```python
from build123d import *

# Parameters (mm, degrees)
BOSS_EXTRU_1_DEPTH      = 50
ESQUISSE3_R             = 25
BOSS_EXTRU_2_DEPTH      = 10
ESQUISSE4_R             = 25
BOSS_EXTRU_3_DEPTH      = 15
COQUE2_START            = 3
COQUE2_DEPTH            = 44
ESQUISSE6_R             = 2.5
ENL_V_MAT_EXTRU_1_DEPTH = 109.272397717


with BuildPart() as part:
    # Esquisse1 → Boss.-Extru.1 (new body)
    with BuildSketch(Plane.XY):
        Polygon((-31.809910954, -22.428852102), (-16.234936413, -34.975571516), (33.765063587, -34.975571516), (62.690506023, -0.503571576), (54.008097139, 48.736816075), (33.432510355, 62.937000175), (-31.809910954, 37.571147898), align=None)
    extrude(amount=BOSS_EXTRU_1_DEPTH)

    # Esquisse3 → Boss.-Extru.2 (add)
    with BuildSketch(Plane(origin=(60.714040151, 10.705523386, 0), x_dir=(0, 0, -1), z_dir=(0.9848077530122085, 0.17364817766692822, 0))):
        with Locations(Location((-25, 13.61798668, 0), (0, 0, 90))):
            Circle(ESQUISSE3_R)
    extrude(amount=BOSS_EXTRU_2_DEPTH)

    # Esquisse4 → Boss.-Extru.3 (add, symmetric)
    with BuildSketch(Plane.ZY.offset(31.809910954)):
        with Locations((25, -3.702211809)):
            Circle(ESQUISSE4_R)
    extrude(amount=BOSS_EXTRU_3_DEPTH, both=True)

    # Coque2: read off the stored shape, not the designer's step
    # Coque2 outline → Coque2 (cut)
    with BuildSketch(Plane.XY.offset(COQUE2_START)):
        Polygon((-28.809910954, 38.737529453), (-28.809910954, -20.993225887), (-11.452809865, -34.975571516), (33.765063587, -34.975571516), (60.173207129, -3.503571576), (55.394878322, 23.595677716), (50.539748489, 51.130487267), (33.432510355, 62.937000175), align=None)
    extrude(amount=COQUE2_DEPTH, mode=Mode.SUBTRACT)

    # Coque2 2: loft between two sections, ruled curve by curve
    coque2_2_from = [
        Edge.make_three_point_arc((68.197379111, 25.853104026, 3), (72.01763902, 4.18733346, 25), (68.197379111, 25.853104026, 47)),
        Edge.make_three_point_arc((68.197379111, 25.853104026, 47), (64.377119202, 47.518874592, 25), (68.197379111, 25.853104026, 3)),
    ]
    coque2_2_to = [
        Edge.make_three_point_arc((55.394878322, 23.595677716, 3), (59.21513823, 1.92990715, 25), (55.394878322, 23.595677716, 47)),
        Edge.make_three_point_arc((55.394878322, 23.595677716, 47), (51.574618413, 45.261448283, 25), (55.394878322, 23.595677716, 3)),
    ]
    coque2_2 = Solid(Shell([*[Face.make_surface_from_curves(coque2_2_from[k], coque2_2_to[k]) for k in range(2)], Face(Wire(coque2_2_from)), Face(Wire(coque2_2_to))]))
    add(coque2_2, mode=Mode.SUBTRACT)

    # Coque2 3: loft between two sections, ruled curve by curve
    coque2_3_from = [
        Edge.make_three_point_arc((-46.809910954, -3.702211809, 47), (-46.809910954, -25.702211809, 25), (-46.809910954, -3.702211809, 3)),
        Edge.make_three_point_arc((-46.809910954, -3.702211809, 3), (-46.809910954, 18.297788191, 25), (-46.809910954, -3.702211809, 47)),
    ]
    coque2_3_to = [
        Edge.make_three_point_arc((-22.947653862, -3.702211809, 47), (-22.947653862, -25.702211809, 25), (-22.947653862, -3.702211809, 3)),
        Edge.make_three_point_arc((-22.947653862, -3.702211809, 3), (-22.947653862, 18.297788191, 25), (-22.947653862, -3.702211809, 47)),
    ]
    coque2_3 = Solid(Shell([*[Face.make_surface_from_curves(coque2_3_from[k], coque2_3_to[k]) for k in range(2)], Face(Wire(coque2_3_from)), Face(Wire(coque2_3_to))]))
    add(coque2_3, mode=Mode.SUBTRACT)

    # Esquisse6 → Enlèv. mat.-Extru.1 (cut, through all)
    with BuildSketch(Plane.XY.offset(50)):
        with Locations((23.91500674, -9.499973142)):
            Circle(ESQUISSE6_R)
    extrude(amount=-ENL_V_MAT_EXTRU_1_DEPTH, mode=Mode.SUBTRACT)


solid = part.part
```
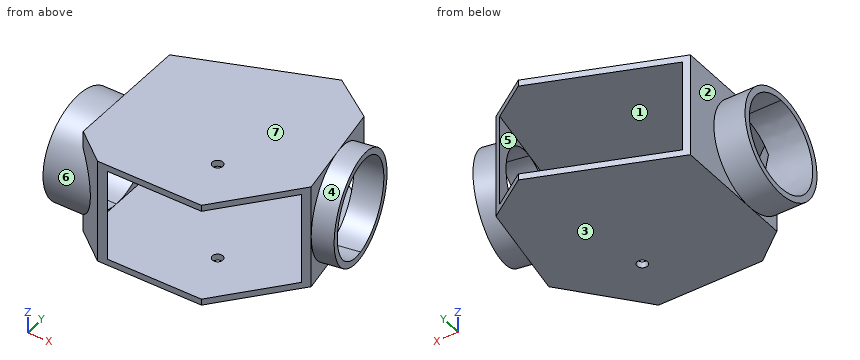
Here's how the part is built. I have some questions about the finished solid (model axes, mm). Face numbers are marked on the shaded views. A direction names the side the tool comes from. Round coordinates to 2 decimals unless told otherwise and drop trailing zeros. Order: outer loops, then holes, each group sorted by start corner. A loop starts at its lowest first (then second) coordinate and runs counter-clockwise, first axis right, second up. Notation, with made-up numbers: M -11.5,38 L 10.5,38 A20 cw 10.5,43 Z; hole C -16.75,-36 d8. An arc over 180 degrees is marked long. One line per question, with ' | ' between items.
1) I need wall thicknesses on line 1 along Z through (x, y) = (4, 6); line 2 along X through (y, z) = (32, 5); line 3 along X through (y, z) = (-1.5, 30). Which ranges of each line are inside material? Lowest first, please.
Working result:
line 1: 0 to 3, 47 to 50 | line 2: -31.81 to -28.81 | line 3: 59.82 to 61.85
2) For the marked faces 5, 6 and 7, which set-ups out of +Z, -Z, +X, -X, +Y, -Y let a thin tool reach every point of the face, with its end or its side?
Working result:
face 5: -Y | face 6: -X | face 7: +Z, +X, -X, +Y, -Y
3) I want a section at B-B, the plane y = 57.5. Write out the boundary of the cut face in (x, z).
Working result:
outline: M 19.45,0 L 41.31,0 L 41.31,3 L 19.45,3 Z; M 19.45,47 L 41.31,47 L 41.31,50 L 19.45,50 Z
4) For pin 1 Ø8 at (y, z) = (-21.5, 17.5) entering from +X; pin 2 Ø3 at (x, y) = (23.92, -9.5) entering from +Z; pin 3 Ø5 at (y, z) = (-23.5, 39.5) entering from +X; pin 4 Ø10 at (y, z) = (3, 33) entering from +X, each with a flat end and sliding along its axis, tell me the tip position at first contact or that it passes through.
Working result:
pin 1: x = -23.22 | pin 2: through | pin 3: x = -22.59 | pin 4: x = 72.5
5) If we mould it in two halves opening along X, with no side actions, what happens to the marked faces 1, 2, 3 and 4? For each: +X half, -X half, draft (parallel to the pull), parting line (faces both ways), or undercut.
Working result:
face 1: undercut | face 2: -X half | face 3: draft | face 4: undercut
6) I want a section at A-A, the plane x = 6. Write out the boundary of the cut face in (y, z), then the cut area to 3 significant figures.
Working result:
outline: M -34.98,0 L 52.27,0 L 52.27,3 L -34.98,3 Z; M -34.98,47 L 52.27,47 L 52.27,50 L -34.98,50 Z | area: 523 mm²
7) I want a section at C-C, the plane z = 31. State how many separate pieces and enclosed holes the cut face has, then the cut area to 3 significant figures.
Working result:
separate pieces: 4 | enclosed holes: 0 | area: 312 mm²
